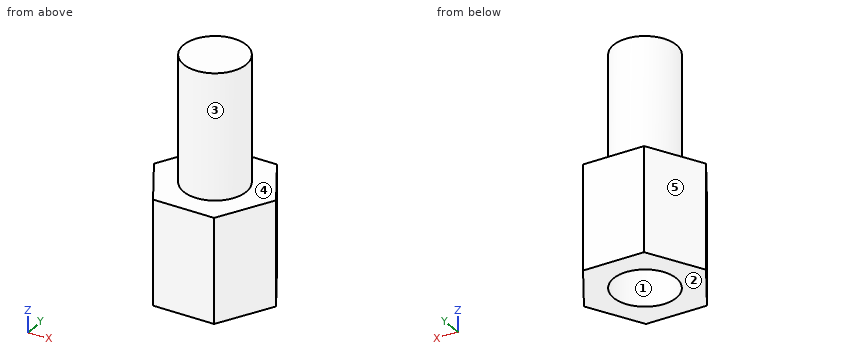
Autodesk Inventor part; units mm, degrees
ref_plane "YZ Plane" through (0, 0, 0) normal (1, 0, 0) x (0, 1, 0)
ref_plane "XZ Plane" through (0, 0, 0) normal (0, 1, 0) x (-1, 0, 0)
ref_plane "XY Plane" through (0, 0, 0) normal (0, 0, 1) x (1, 0, 0)
sketch "Sketch1" plane through (0, 0, 0) normal (0, 0, 1) x (1, 0, 0)
  line L0 (2.8868, 0) -> (1.4434, -2.5)
  line L1 (1.4434, -2.5) -> (-1.4434, -2.5)
  line L2 (-1.4434, -2.5) -> (-2.8868, 0)
  line L3 (-2.8868, 0) -> (-1.4434, 2.5)
  line L4 (-1.4434, 2.5) -> (1.4434, 2.5)
  line L5 (1.4434, 2.5) -> (2.8868, 0)
  point P0 (0, 0)
  point P1 (0, 0)
  dimension "d0" = 5
extrude "Extrusion1" add sketch "Sketch1" along normal blind 5
sketch "Sketch2" plane through (0, 0, 5) normal (0, 0, 1) x (1, 0, 0)
  circle A0 centre (0, 0) radius 1.5
  dimension "d3" = 3
extrude "Extrusion2" add sketch "Sketch2" along normal blind 6
sketch "Sketch3" plane through (0, 0, 0) normal (0, 0, -1) x (-1, 0, 0)
  circle A0 centre (0, 0) radius 1.5
  dimension "d6" = 3
extrude "Extrusion3" cut sketch "Sketch3" against normal blind 4
properties part number "Spacer7mm_m3"
Could you check a few things on this model? Use its own coordinates, in mm. Face numbers are marked on the shaded views. A direction names the side the tool comes from. Coordinates: 2 decimals unless noted, no trailing zeros. Order: outer loops, then holes, each group sorted by start corner. A loop starts at its lowest first (then second) coordinate and runs counter-clockwise, first axis right, second up. Notation, with made-up numbers: (73, 43.25) -> (92, 43.25) arc R11 cw to (92, 50.25) -> close; hole circle Ø7 at (-36, -10.5). An arc over 180 degrees is marked (long way). One line per item, written item: value. Start each with the question number.
1) Imagine slicing it at D-D on x = 1.95. List the corners of the cut face in (y, z) for me.
2) I'm going to push flat-ended pins straight in: pin 1 (1 mm diameter, centred on y = 0.5, z = 8, fed in from -X); pin 2 (0.9 mm diameter, centred on x = 0, y = 0.5, fed in from -Z); pin 3 (1 mm diameter, centred on x = -2, z = 4, fed in from +Y). Where does each tip first touch, or does it pass through?
3) If I drill on L1, parallel to Y at x = 0, z = 3.25; L2, parallel to Z at x = -1.3, y = 0.4; L3, parallel to Y at x = 0.85, z = 2.25, over which ranges is the centre line in solid material (lowest first)? Write a range as [from, to].
4) Imagine slicing it at A-A on x = 0. List the corners of the cut face in (y, z) for me.
5) Which directions (+Z, -Z, +X, -X, +Y, -Y) give clear straight access to the entire face, cutting with the end or side of a thin tool? Please do the marked faces 4 and 5.
6) Imagine slicing it at B-B on y = 1. List the corners of the cut face in (x, z) for me, plus the area to 3 significant figures.
7) Imagine slicing it at C-C on z = 4.5. List the corners of the cut face in (x, y) for me.
8) We'd pull the mould along X, two halves only. Please class the marked faces 1, 2 and 3: +X half, -X half, draft (parallel to the pull), parting line (faces both ways), or undercut.
Answer list:
1. outline: (-1.62, 0) -> (1.62, 0) -> (1.62, 5) -> (-1.62, 5) -> close
2. pin 1: stops at x = -1.5
2. pin 2: stops at z = 4
2. pin 3: stops at y = 2.4
3. L1: y = [-2.5, -1.5], [1.5, 2.5]
3. L2: z = [4, 11]
3. L3: y = [-2.5, -1.24], [1.24, 2.5]
4. outline: (-2.5, 0) -> (-1.5, 0) -> (-1.5, 4) -> (1.5, 4) -> (1.5, 0) -> (2.5, 0) -> (2.5, 5) -> (1.5, 5) -> (1.5, 11) -> (-1.5, 11) -> (-1.5, 5) -> (-2.5, 5) -> close
5. face 4: +Z
5. face 5: +Z, -Z, -X, +Y
6. outline: (-2.31, 0) -> (-1.12, 0) -> (-1.12, 4) -> (1.12, 4) -> (1.12, 0) -> (2.31, 0) -> (2.31, 5) -> (1.12, 5) -> (1.12, 11) -> (-1.12, 11) -> (-1.12, 5) -> (-2.31, 5) -> close
6. area: 27.6 mm2
7. outline: (-2.89, 0) -> (-1.44, -2.5) -> (1.44, -2.5) -> (2.89, 0) -> (1.44, 2.5) -> (-1.44, 2.5) -> close
8. face 1: undercut
8. face 2: draft
8. face 3: parting line
